from build123d import *

# Parameters (mm, degrees)
SKETCH1_R          = 3.175
EXTRUDE1_DEPTH     = 127
CHAMFER3_SIZE      = 0.9525
SKETCH6_R          = 4.7625
EXTRUDE2_DEPTH     = 6.35
CUT_EXTRUDE1_DEPTH = 3.571875
CHAMFER1_SIZE      = 0.47625
CHAMFER2_SIZE      = 0.238125


with BuildPart() as part:
    # Sketch1 → Extrude1 (new body)
    with BuildSketch(Plane.XY):
        Circle(SKETCH1_R)
    extrude(amount=-EXTRUDE1_DEPTH)

    # Chamfer3
    chamfer3_edges = [part.edges().sort_by_distance(p)[0] for p in [
        (-3.175, 0, 0),
    ]]
    chamfer(chamfer3_edges, length=CHAMFER3_SIZE)

    # Sketch6 → Extrude2 (add)
    with BuildSketch(Plane(origin=(0, 0, -127), x_dir=(-1, 0, 0), z_dir=(0, 0, -1))):
        Circle(SKETCH6_R)
    extrude(amount=EXTRUDE2_DEPTH)

    # Sketch7 → Cut-Extrude1 (cut)
    with BuildSketch(Plane(origin=(0, 0, -133.35), x_dir=(-1, 0, 0), z_dir=(0, 0, -1))):
        Polygon((0, 2.749630657), (-2.38125, 1.374815329), (-2.38125, -1.374815329), (0, -2.749630657), (2.38125, -1.374815329), (2.38125, 1.374815329), align=None)
    extrude(amount=-CUT_EXTRUDE1_DEPTH, mode=Mode.SUBTRACT)

    # Cut-Extrude2 cone 1 section (through the dimple's axis) → Cut-Extrude2 (revolve, cut)
    with BuildSketch(Plane(origin=(0, 0, -133.35), x_dir=(0, 1, 0), z_dir=(1, 0, 0))):
        Polygon((0, 0), (2.749630657, 0), (0, 2.749630657), align=None)
    revolve(axis=Axis((0, 0, -133.35), (0, 0, 1)), mode=Mode.SUBTRACT)

    # Chamfer1
    chamfer1_edges = [part.edges().sort_by_distance(p)[0] for p in [
        (4.7625, 0, -133.35),
    ]]
    chamfer(chamfer1_edges, length=CHAMFER1_SIZE)

    # Chamfer2
    chamfer2_edges = [part.edges().sort_by_distance(p)[0] for p in [
        (4.7625, 0, -127),
    ]]
    chamfer(chamfer2_edges, length=CHAMFER2_SIZE)


solid = part.part
Verification items for the finished model (mm, model axes). A direction names the side the tool comes from. Coordinates: 2 decimals unless noted, no trailing zeros. Order: outer loops, then holes, each group sorted by start corner. A loop starts at its lowest first (then second) coordinate and runs counter-clockwise, first axis right, second up.
1. Set-up check for faces 5 (the face through (1.21, -2.05, -131.59)), 6 (the face through (0, 0, 0)): record each of +Z, -Z, +X, -X, +Y, -Y from which the full face is reachable in a straight line by a thin tool's end or side.
Results found:
face 5: -Z
face 6: +Z, +X, -X, +Y, -Y
2. Scan lines: line 1 (Z direction, x = -2, y = -3.5); line 2 (Z direction, x = 1, y = -2); line 3 (Y direction, x = -0.25, z = -126). Record each from-to range of solid material in increasing order.
Results found:
line 1: z = -133.35 to -127
line 2: z = -129.78 to -0.01
line 3: y = -3.17 to 3.17
3. Go/stop test with flat-tipped pins: pin 1 Ø4 at (y, z) = (-2.5, -71) entering from -X; pin 2 Ø3 at (x, y) = (-2, 0.5) entering from -Z; pin 3 Ø1.4 at (x, y) = (-0.5, -1) entering from -Z; pin 4 Ø4 at (x, z) = (0, -92.5) entering from +Y (3 decimals). Record where each tip stops, or that it passes through.
Results found:
pin 1: stops at x = -3.14
pin 2: stops at z = -133.35
pin 3: stops at z = -129.78
pin 4: stops at y = 3.175
4. Release check for a two-part mould opening along Y. For faces 1 (the face through (-1.21, 2.05, -131.59)), 2 (the face through (-0.69, -3.1, -63.09)), 3 (the face through (1.174, 2.072, -131.589)), 4 (the face through (-2, -3, -127)) record: +Y half, -Y half, draft (parallel to the pull), parting line (faces both ways), or undercut.
Results found:
face 1: undercut
face 2: parting line
face 3: undercut
face 4: draft
5. Sectioned sample at B-B, the plane z = -124.5. Record the cut outline in (x, y) (3 decimals), and give its area (3 significant figures).
Results found:
outline: circle Ø6.35 at (0, 0)
area: 31.7 mm2
